Read the model definition and answer for the solid it produces. Units are mm, in the model's axes. Coordinates: 2 decimals unless noted, no trailing zeros. Use one line per item in the form item = value. Start each with the question number.
1) Consider line 1 (Z direction, x = 0, y = -4.25); line 2 (Z direction, x = 0, y = -5.75); line 3 (X direction, y = -0.5, z = 8). Determine where each line is inside the solid, lowest interval first.
2) A cutting plane is placed at A-A (x = 0). State how many separate pieces and enclosed holes the cut face has, and give its area (3 significant figures).
3) Each of these flat-tipped pins is pushed along its axis until it touches: P1, Ø4.5, axis at y = -2.5, z = 27, coming from the -X side; P2, Ø4, axis at y = -5.5, z = -3.5, coming from the -X side; P3, Ø1.6, axis at x = 0, z = 95, coming from the +Y side. Where does it stop, or does it pass through?
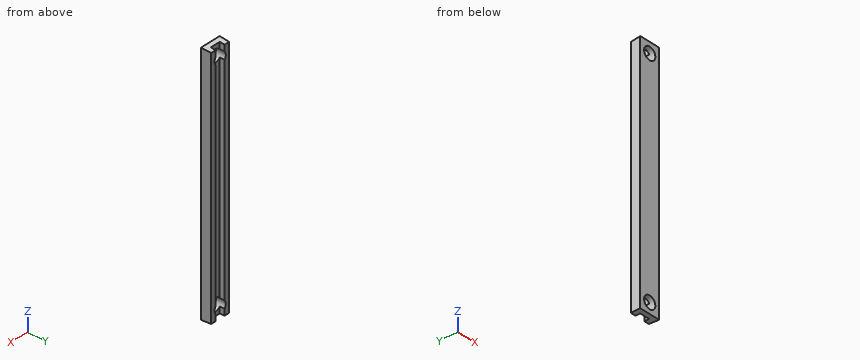
from build123d import *

# Parameters (mm, degrees)
F0_W     = 16
F0_H     = 196
F1_DEPTH = 8
F1_TAPER = -3
F2_W     = 8
F2_H     = 200
F3_DEPTH = 4
F4_R     = 5
F5_DEPTH = 25.4


with BuildPart() as f1:
    # F0 (on Front) → F1 (new body)
    with BuildSketch(Plane.XZ):
        Rectangle(F0_W, F0_H)
    extrude(amount=F1_DEPTH, taper=F1_TAPER)

    # F2 (on face) → F3 (cut)
    with BuildSketch(Plane.XZ):
        Rectangle(F2_W, F2_H)
    extrude(amount=F3_DEPTH, mode=Mode.SUBTRACT)

    # F4 (on Front) → F5 (cut)
    with BuildSketch(Plane.XZ):
        with Locations((0, 90)):
            Circle(F4_R)
        with Locations((0, -90)):
            Circle(F4_R)
    extrude(amount=F5_DEPTH, mode=Mode.SUBTRACT)


solid = f1.part
Found:
q1.line_1 = -98.22 to -95, -85 to 85, 95 to 98.22
q1.line_2 = -98.3 to -95, -85 to 85, 95 to 98.3
q1.line_3 = -8.03 to -4, 4 to 8.03
q2.separate_pieces = 3
q2.enclosed_holes = 0
q2.area = 707 mm^2
q3.P1 = -8.25
q3.P2 = -8.39
q3.P3 = -4
